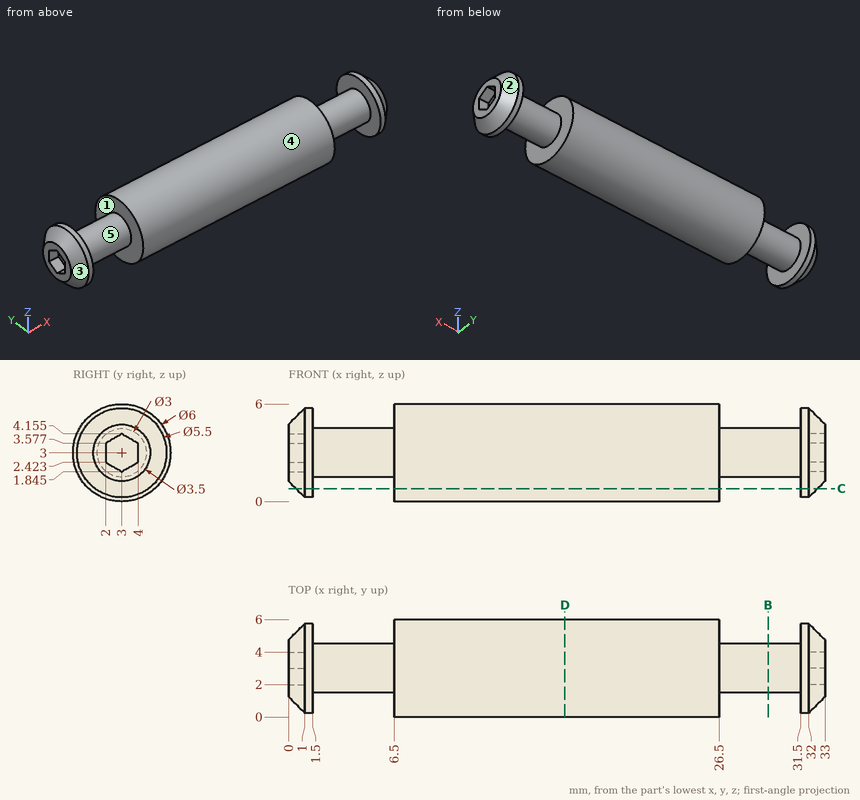
Print and shaded views of the part. All mm, measured from the part's lowest x, y and z. A direction names the side the tool comes from. Give positions to 0.01 mm unless a question says otherwise; leave off trailing zeros. Write each loop counter-clockwise with the first axis right and the second up, starting at its lowest first coordinate (ties: lowest second). Pieces come first, ordered by that corner, then holes. Notation, with made-up numbers: (62, -1) - (116, -1) arc R7 cw to (116, 12) - close; hole circle Ø11 at (0, 63). An arc over 180 degrees is marked (long way). One line per question, with ' | ' between items. Start each with the question number.
(1) 3-axis set-ups, long thin cutter, end or side, ignore diameter. For the marked faces 1 and 2: which of +Z, -Z, +X, -X, +Y, -Y reach the whole face in a straight line?
(2) Slice it at B-B on x = 29.5. Write the cut outline in (y, z).
(3) Slice it at D-D on x = 17. Write the cut outline in (y, z).
(4) Slice it at C-C on z = 0.8. Give the number of separate pieces and of enclosed holes in the cut face.
(5) Two-plate mould, pull along X, no slides. Class the marked faces 3, 4 and 5: +X half, -X half, draft (parallel to the pull), parting line (faces both ways), or undercut.
(6) Pin check, flat tips, straight feed: P1, Ø3, axis at y = 1.5, z = 2, coming from the +X side; P2, Ø0.5, axis at x = 32.5, z = 3, coming from the +Y side; P3, Ø1, axis at y = 3, z = 3, coming from the -X side; P4, Ø0.8, axis at x = 32.5, z = 3, coming from the -Y side. Stop position of each tip, or through.
(7) Wall check: line 1 along X through (y, z) = (4.55, 3.3); line 2 along X through (y, z) = (5.6, 2.9); line 3 along Y through (x, z) = (8.5, 2.9). Give the ranges that are in metal, low to high. Write a range as from..to.
Results below:
1) face 1: none | face 2: +X
2) outline: circle Ø3 at (3, 3)
3) outline: circle Ø6 at (3, 3)
4) separate pieces: 3 | enclosed holes: 0
5) face 3: -X half | face 4: draft | face 5: undercut
6) P1: x = 33 | P2: y = 5.5 | P3: x = 1 | P4: y = 0.35
7) line 1: 0..1.5, 6.5..26.5, 31.5..33 | line 2: 0.85..1.5, 6.5..26.5, 31.5..32.15 | line 3: 0..6
